Work out the finished part from the listing and answer in its coordinate system (mm). A direction names the side the tool comes from. Coordinates: 2 decimals unless noted, no trailing zeros. Order: outer loops, then holes, each group sorted by start corner. A loop starts at its lowest first (then second) coordinate and runs counter-clockwise, first axis right, second up. Notation, with made-up numbers: M 51.5,22 L 55.5,22 A19 cw 55.5,59 Z; hole C -31.5,-2 d7. An arc over 180 degrees is marked long. Use a Markdown table: item, result.
from build123d import *

# Parameters (mm, degrees)
F0_W     = 100
F0_H     = 100
F1_DEPTH = 25
F2_W     = 90
F2_H     = 90
F3_DEPTH = 10
F4_R     = 10


with BuildPart() as f1:
    # F0 (on Top) → F1 (new body)
    with BuildSketch(Plane.XY):
        Rectangle(F0_W, F0_H)
    extrude(amount=F1_DEPTH)

    # F2 (on face) → F3 (cut)
    with BuildSketch(Plane.XY.offset(25)):
        Rectangle(F2_W, F2_H)
    extrude(amount=-F3_DEPTH, mode=Mode.SUBTRACT)

    # F4
    f4_edges = [f1.edges().sort_by_distance(p)[0] for p in [
        (50, 50, 12.5),
        (45, 45, 20),
        (-45, 45, 20),
        (-50, 50, 12.5),
        (-50, -50, 12.5),
        (-45, -45, 20),
        (50, -50, 12.5),
        (45, -45, 20),
    ]]
    fillet(f4_edges, radius=F4_R)


solid = f1.part
(1) Determine the mould class of faces 3 (the cylindrical face through (-47.15, 46.99, 12.68)), 4 (the cylindrical face through (-41.99, 42.15, 19.93)), 5 (the flat face through (-1, 50, 12)) for opening direction X: pulls with the +X half, pulls with the -X half, needs draft (parallel to the pull), parting line crosses it, or undercut.
Conclusion:
| item | result |
|---|---|
| face 3 | pulls with the -X half |
| face 4 | undercut |
| face 5 | needs draft |
(2) A cutting plane is placed at A-A (x = -20.5). Determine the outline of the cut face in (y, z), then the cut area to 3 significant figures.
Conclusion:
| item | result |
|---|---|
| outline | M -50,0 L 50,0 L 50,25 L 45,25 L 45,15 L -45,15 L -45,25 L -50,25 Z |
| area | 1,600 mm2 |
(3) Which of the six approach directions +Z, -Z, +X, -X, +Y, -Y give full straight-line access (tool end or side, diameter ignored) to faces 1 (the flat face through (45, 0, 20)), 2 (the flat face through (-1, 1, 0))?
Conclusion:
| item | result |
|---|---|
| face 1 | +Z |
| face 2 | -Z, +X, -X, +Y, -Y |
(4) A cutting plane is placed at B-B (z = 21.5). Determine the outline of the cut face in (x, y).
Conclusion:
| item | result |
|---|---|
| outline | M -50,-40 A10 ccw -40,-50 L 40,-50 A10 ccw 50,-40 L 50,40 A10 ccw 40,50 L -40,50 A10 ccw -50,40 Z; hole M -45,-35 A10 ccw -35,-45 L 35,-45 A10 ccw 45,-35 L 45,35 A10 ccw 35,45 L -35,45 A10 ccw -45,35 Z |
(5) Straight lines are drawn through the part: L1, parallel to X at y = -19, z = 22; L2, parallel to Z at x = 36, y = 12. For each, find the intervals that lie inside material, in ascending order.
Conclusion:
| item | result |
|---|---|
| L1 | -50 to -45, 45 to 50 |
| L2 | 0 to 15 |
(6) Given P1, Ø10, axis at x = -35, y = 14, coming from the -Z side, flat-ended and moving along its own axis, determine where the tip first touches the part or whether it passes through.
Conclusion:
| item | result |
|---|---|
| P1 | z = 0 |
